Geometry: final body of the model. Coordinates: model frame, mm. Face numbers are marked on the shaded views. A direction names the side the tool comes from. Give positions to 0.01 mm unless a question says otherwise; leave off trailing zeros. Loops run counter-clockwise (first coordinate to the right, second up) from the corner with the lowest first, then second, coordinate; pieces in that order, holes last.
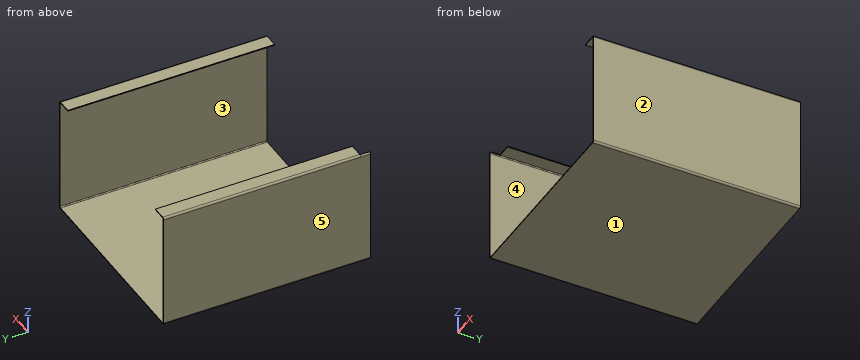
from build123d import *

# Parameters (mm, degrees)
BASE_FLANGE1_DEPTH     = 0.6
SKETCHED_BEND1_DEPTH   = 148
SKETCHED_START         = 7
SKETCHED_BEND1_2_DEPTH = 141
SKETCHED_BEND1_3_DEPTH = 7


# Read off the part's stored shape, not the designer's step: Sketched Bend1
# Sheet-metal steps are written as plain solids
with BuildPart() as part:
    # Sketch1 → Base-Flange1 (new body)
    with BuildSketch(Plane.XY):
        Polygon((0, 7), (10, 7), (10, 0), (326, 0), (326, 148), (0, 148), align=None)
    extrude(amount=BASE_FLANGE1_DEPTH)

    # Sketched Bend1 outline → Sketched Bend1 (cut)
    with BuildSketch(Plane(origin=(0, 0, 0), x_dir=(1, 0, 0), z_dir=(0, 1, 0))):
        with BuildLine():
            ThreePointArc((93.221288384, -0.6), (93.703370184, -0.159519051), (94.3366, 0))
            Line((94.3366, 0), (0, 0))
            Line((0, 0), (0, -0.6))
            Line((0, -0.6), (93.221288384, -0.6))
        make_face()
        with BuildLine():
            ThreePointArc((231.6634, 0), (232.296629816, -0.159519051), (232.778711616, -0.6))
            Line((232.778711616, -0.6), (326, -0.6))
            Line((326, -0.6), (326, 0))
            Line((326, 0), (231.6634, 0))
        make_face()
    extrude(amount=SKETCHED_BEND1_DEPTH, mode=Mode.SUBTRACT)

    # Sketched Bend1 2 outline → Sketched Bend1 2 (add)
    with BuildSketch(Plane(origin=(0, 0, 0), x_dir=(1, 0, 0), z_dir=(0, 1, 0)).offset(SKETCHED_START)):
        with BuildLine():
            Line((93.6, -82.708312528), (93.6, -1.3366))
            ThreePointArc((93.6, -1.3366), (93.815745145, -0.815745145), (94.3366, -0.6))
            Line((94.3366, -0.6), (93.221288384, -0.6))
            ThreePointArc((93.221288384, -0.6), (93.056516982, -0.952039176), (93, -1.3366))
            Line((93, -1.3366), (93, -82.708312528))
            ThreePointArc((93, -82.708312528), (93.391481076, -83.653431451), (94.3366, -84.044912528))
            Line((94.3366, -84.044912528), (104.044912528, -84.044912528))
            Line((104.044912528, -84.044912528), (104.044912528, -83.444912528))
            Line((104.044912528, -83.444912528), (94.3366, -83.444912528))
            ThreePointArc((94.3366, -83.444912528), (93.815745145, -83.229167383), (93.6, -82.708312528))
        make_face()
        with BuildLine():
            Line((232.778711616, -0.6), (231.6634, -0.6))
            ThreePointArc((231.6634, -0.6), (232.184254855, -0.815745145), (232.4, -1.3366))
            Line((232.4, -1.3366), (232.4, -82.708312528))
            ThreePointArc((232.4, -82.708312528), (232.184254855, -83.229167383), (231.6634, -83.444912528))
            Line((231.6634, -83.444912528), (221.955087472, -83.444912528))
            Line((221.955087472, -83.444912528), (221.955087472, -84.044912528))
            Line((221.955087472, -84.044912528), (231.6634, -84.044912528))
            ThreePointArc((231.6634, -84.044912528), (232.608518924, -83.653431451), (233, -82.708312528))
            Line((233, -82.708312528), (233, -1.3366))
            ThreePointArc((233, -1.3366), (232.943483018, -0.952039176), (232.778711616, -0.6))
        make_face()
    extrude(amount=SKETCHED_BEND1_2_DEPTH)

    # Sketched Bend1 3 outline → Sketched Bend1 3 (add)
    with BuildSketch(Plane(origin=(0, 0, 0), x_dir=(1, 0, 0), z_dir=(0, 1, 0))):
        with BuildLine():
            Line((93.6, -82.708312528), (93.6, -1.3366))
            ThreePointArc((93.6, -1.3366), (93.815745145, -0.815745145), (94.3366, -0.6))
            Line((94.3366, -0.6), (93.221288384, -0.6))
            ThreePointArc((93.221288384, -0.6), (93.056516982, -0.952039176), (93, -1.3366))
            Line((93, -1.3366), (93, -82.708312528))
            ThreePointArc((93, -82.708312528), (93.268285315, -83.511558003), (93.965439614, -83.992345054))
            Line((93.965439614, -83.992345054), (94.132053583, -83.415942603))
            ThreePointArc((94.132053583, -83.415942603), (93.747851985, -83.150980953), (93.6, -82.708312528))
        make_face()
        with BuildLine():
            Line((232.778711616, -0.6), (231.6634, -0.6))
            ThreePointArc((231.6634, -0.6), (232.184254855, -0.815745145), (232.4, -1.3366))
            Line((232.4, -1.3366), (232.4, -82.708312528))
            ThreePointArc((232.4, -82.708312528), (232.184254855, -83.229167383), (231.6634, -83.444912528))
            Line((231.6634, -83.444912528), (221.955087472, -83.444912528))
            Line((221.955087472, -83.444912528), (221.955087472, -84.044912528))
            Line((221.955087472, -84.044912528), (231.6634, -84.044912528))
            ThreePointArc((231.6634, -84.044912528), (232.608518924, -83.653431451), (233, -82.708312528))
            Line((233, -82.708312528), (233, -1.3366))
            ThreePointArc((233, -1.3366), (232.943483018, -0.952039176), (232.778711616, -0.6))
        make_face()
    extrude(amount=SKETCHED_BEND1_3_DEPTH)


solid = part.part
Item 1: Section query C-C on y = 90.5. Return loops of the section in (x, z).
Values follow:
outline: (93, 1.34) arc R1.34 ccw to (94.34, 0) - (231.66, 0) arc R1.34 ccw to (233, 1.34) - (233, 82.71) arc R1.34 ccw to (231.66, 84.04) - (221.96, 84.04) - (221.96, 83.44) - (231.66, 83.44) arc R0.74 cw to (232.4, 82.71) - (232.4, 1.34) arc R0.74 cw to (231.66, 0.6) - (94.34, 0.6) arc R0.74 cw to (93.6, 1.34) - (93.6, 82.71) arc R0.74 cw to (94.34, 83.44) - (104.04, 83.44) - (104.04, 84.04) - (94.34, 84.04) arc R1.34 ccw to (93, 82.71) - close
Item 2: Ray query, probe 1 along X at (y, z) = (140, 77.5); probe 2 along Z at (x, y) = (104, 74.5); probe 3 along Z at (x, y) = (132.5, 31.5). Return the intervals inside material, ascending.
Values follow:
probe 1: x = 93 to 93.6, 232.4 to 233
probe 2: z = 0 to 0.6, 83.44 to 84.04
probe 3: z = 0 to 0.6
Item 3: Set-up query: the marked faces 4 and 5. Return all of +Z, -Z, +X, -X, +Y, -Y with unobstructed straight access to the full face (end or side cutting, diameter ignored); none if empty.
Values follow:
face 4: +Y, -Y
face 5: +Z, -Z, -X, +Y, -Y
Item 4: Section query B-B on x = 224.5. Return loops of the section in (y, z).
Values follow:
outline: (0, 0) - (148, 0) - (148, 0.6) - (0, 0.6) - close; (0, 83.44) - (148, 83.44) - (148, 84.04) - (0, 84.04) - close
Item 5: Draft query along Z for the marked faces 1, 2 and 3. Return one class per face: +Z half, -Z half, draft (parallel to the pull), parting line (faces both ways), or undercut.
Values follow:
face 1: -Z half
face 2: draft
face 3: undercut
Item 6: Pin query (flat end, axial travel): pin 1 (10 mm diameter, centred on x = 199.5, y = 33, fed in from +Z); pin 2 (0.5 mm diameter, centred on x = 100.5, z = 84, fed in from -Y); pin 3 (0.7 mm diameter, centred on y = 73, z = 83.5, fed in from +X). Return the tip coordinate at first contact, or that it passes through.
Values follow:
pin 1: stops at z = 0.6
pin 2: stops at y = 7
pin 3: stops at x = 232.92
Item 7: Section query A-A on z = 76. Return loops of the section in (x, y), plus the area to 3 significant figures.
Values follow:
outline: (93, 0) - (93.6, 0) - (93.6, 148) - (93, 148) - close; (232.4, 0) - (233, 0) - (233, 148) - (232.4, 148) - close
area: 178 mm2
